from build123d import *

# Parameters (mm, degrees)
BOSS_EXTRU_1_DEPTH      = 23
ENL_V_MAT_EXTRU_1_DEPTH = 21.5
ESQUISSE3_W             = 8.5
ESQUISSE3_H             = 8.4
BOSS_EXTRU_3_DEPTH      = 3.4
BOSS_EXTRU_5_REACH      = 9.309
ESQUISSE4_W             = 1.5
ESQUISSE4_H             = 3.406602833
ESQUISSE23_R            = 1.15
ENL_V_MAT_EXTRU_2_DEPTH = 4
ESQUISSE24_W            = 7
ESQUISSE24_H            = 8.4
BOSS_EXTRU_6_DEPTH      = 3.4
ENL_V_MAT_EXTRU_4_REACH = 77.809
ESQUISSE26_W            = 15.35
ESQUISSE26_H            = 16.4
ESQUISSE27_W            = 1
ESQUISSE27_H            = 17
BOSS_EXTRU_7_DEPTH      = 4
CHANFREIN1_SIZE         = 2
ENL_V_MAT_EXTRU_5_REACH = 76
ESQUISSE28_W            = 4.2
ESQUISSE28_H            = 11.5
ENL_V_MAT_EXTRU_6_REACH = 76
ESQUISSE29_W            = 4.2
ESQUISSE29_H            = 8.5
ESQUISSE30_W            = 13
ESQUISSE30_H            = 4.2
ENL_V_MAT_EXTRU_8_DEPTH = 4
CONG_1_R                = 2


with BuildPart() as part:
    # Esquisse1 → Boss.-Extru.1 (new body)
    with BuildSketch(Plane.XY):
        Polygon((-2.5, -35), (3, -40.809475019), (23, -40.809475019), (28.5, -35), (37, -35), (37, 35), (-37, 35), (-37, -35), align=None)
    extrude(amount=BOSS_EXTRU_1_DEPTH)

    # Esquisse2 → Enlèv. mat.-Extru.1 (cut)
    with BuildSketch(Plane.XY.offset(23)):
        Polygon((-2.5, -33.5), (3, -39.309475019), (23, -39.309475019), (28.5, -33.5), (35.5, -33.5), (35.5, 33.5), (-35.5, 33.5), (-35.5, -33.5), align=None)
    extrude(amount=-ENL_V_MAT_EXTRU_1_DEPTH, mode=Mode.SUBTRACT)

    # Esquisse3 → Boss.-Extru.3 (add)
    with BuildSketch(Plane.XY.offset(1.5)):
        with Locations((31.25, 29.3)):
            Rectangle(ESQUISSE3_W, ESQUISSE3_H)
        with Locations((-31.25, 29.3)):
            Rectangle(ESQUISSE3_W, ESQUISSE3_H)
        with Locations((31.25, -29.3)):
            Rectangle(ESQUISSE3_W, ESQUISSE3_H)
        with Locations((-31.25, -29.3)):
            Rectangle(ESQUISSE3_W, ESQUISSE3_H)
    extrude(amount=BOSS_EXTRU_3_DEPTH)

    # Esquisse4 → Boss.-Extru.5 (add, up to next)
    with BuildSketch(Plane.XZ.offset(33.5), mode=Mode.PRIVATE) as boss_extru_5_sk1:
        with Locations((27.75, 3.196698584)):
            Rectangle(ESQUISSE4_W, ESQUISSE4_H)
    boss_extru_5_tool1 = extrude(boss_extru_5_sk1.sketch, amount=BOSS_EXTRU_5_REACH, mode=Mode.PRIVATE) - part.part
    add(boss_extru_5_tool1.solids().sort_by_distance((27.75, -33.5, 3.196699))[0])

    # Esquisse23 → Enlèv. mat.-Extru.2 (cut)
    with BuildSketch(Plane.XY.offset(4.9)):
        with Locations((31.3, 29.3)):
            Circle(ESQUISSE23_R)
        with Locations((-31.3, 29.3)):
            Circle(ESQUISSE23_R)
        with Locations((31.3, -28.9)):
            Circle(ESQUISSE23_R)
        with Locations((-31.3, -28.9)):
            Circle(ESQUISSE23_R)
    extrude(amount=-ENL_V_MAT_EXTRU_2_DEPTH, mode=Mode.SUBTRACT)

    # Esquisse24 → Boss.-Extru.6 (add)
    with BuildSketch(Plane.XY.offset(1.5)):
        with Locations((-8.3, 29.3)):
            Rectangle(ESQUISSE24_W, ESQUISSE24_H)
        with Locations((-8.3, -29.3)):
            Rectangle(ESQUISSE24_W, ESQUISSE24_H)
    extrude(amount=BOSS_EXTRU_6_DEPTH)

    # Esquisse26 → Enlèv. mat.-Extru.4 (cut, up to next)
    with BuildSketch(Plane.XZ.offset(40.809475019), mode=Mode.PRIVATE) as enl_v_mat_extru_4_sk1:
        with Locations((13, 14.8)):
            Rectangle(ESQUISSE26_W, ESQUISSE26_H)
    enl_v_mat_extru_4_tool1 = extrude(enl_v_mat_extru_4_sk1.sketch, amount=-ENL_V_MAT_EXTRU_4_REACH, mode=Mode.PRIVATE) & part.part
    add(enl_v_mat_extru_4_tool1.solids().sort_by_distance((13, -40.809475, 14.8))[0], mode=Mode.SUBTRACT)

    # Esquisse27 → Boss.-Extru.7 (add)
    with BuildSketch(Plane(origin=(-35.5, 0, 0), x_dir=(0, 0, -1), z_dir=(1, 0, 0))):
        with Locations((-16.9, 3.4)):
            Rectangle(ESQUISSE27_W, ESQUISSE27_H)
    extrude(amount=BOSS_EXTRU_7_DEPTH)

    # Chanfrein1
    chanfrein1_edges = [part.edges().sort_by_distance(p)[0] for p in [
        (-35.5, 3.4, 16.4),
    ]]
    chamfer(chanfrein1_edges, length=CHANFREIN1_SIZE)

    # Esquisse28 → Enlèv. mat.-Extru.5 (cut, up to next)
    with BuildSketch(Plane.ZY.offset(37), mode=Mode.PRIVATE) as enl_v_mat_extru_5_sk1:
        with Locations((20.9, 20.1)):
            Rectangle(ESQUISSE28_W, ESQUISSE28_H)
    enl_v_mat_extru_5_tool1 = extrude(enl_v_mat_extru_5_sk1.sketch, amount=-ENL_V_MAT_EXTRU_5_REACH, mode=Mode.PRIVATE) & part.part
    add(enl_v_mat_extru_5_tool1.solids().sort_by_distance((-37, 20.1, 20.9))[0], mode=Mode.SUBTRACT)

    # Esquisse29 → Enlèv. mat.-Extru.6 (cut, up to next)
    with BuildSketch(Plane.ZY.offset(37), mode=Mode.PRIVATE) as enl_v_mat_extru_6_sk1:
        with Locations((20.9, -8.9)):
            Rectangle(ESQUISSE29_W, ESQUISSE29_H)
    enl_v_mat_extru_6_tool1 = extrude(enl_v_mat_extru_6_sk1.sketch, amount=-ENL_V_MAT_EXTRU_6_REACH, mode=Mode.PRIVATE) & part.part
    add(enl_v_mat_extru_6_tool1.solids().sort_by_distance((-37, -8.9, 20.9))[0], mode=Mode.SUBTRACT)
    # Esquisse29 → Enlèv. mat.-Extru.6 (cut, up to next)
    with BuildSketch(Plane.ZY.offset(37), mode=Mode.PRIVATE) as enl_v_mat_extru_6_sk2:
        with Locations((20.9, -21.5)):
            Rectangle(ESQUISSE29_W, ESQUISSE29_H)
    enl_v_mat_extru_6_tool2 = extrude(enl_v_mat_extru_6_sk2.sketch, amount=-ENL_V_MAT_EXTRU_6_REACH, mode=Mode.PRIVATE) & part.part
    add(enl_v_mat_extru_6_tool2.solids().sort_by_distance((-37, -21.5, 20.9))[0], mode=Mode.SUBTRACT)

    # Esquisse30 → Enlèv. mat.-Extru.8 (cut)
    with BuildSketch(Plane(origin=(0, 35, 0), x_dir=(1, 0, 0), z_dir=(0, 1, 0))):
        with Locations((-17.6, -20.9)):
            Rectangle(ESQUISSE30_W, ESQUISSE30_H)
    extrude(amount=-ENL_V_MAT_EXTRU_8_DEPTH, mode=Mode.SUBTRACT)

    # Congé1
    cong_1_edges = [part.edges().sort_by_distance(p)[0] for p in [
        (28.5, -35, 11.5),
        (23, -40.809475019, 11.5),
        (3, -40.809475019, 11.5),
        (-2.5, -35, 11.5),
        (-37, -35, 11.5),
        (-37, 35, 11.5),
        (37, 35, 11.5),
        (37, -35, 11.5),
        (35.5, 33.5, 13.95),
        (-35.5, 33.5, 13.95),
        (35.5, -33.5, 13.95),
        (-35.5, -33.5, 13.95),
    ]]
    fillet(cong_1_edges, radius=CONG_1_R)


solid = part.part
Could you check a few things on this model? Use its own coordinates, in mm. A direction names the side the tool comes from. Coordinates: 2 decimals unless noted, no trailing zeros. Order: outer loops, then holes, each group sorted by start corner. A loop starts at its lowest first (then second) coordinate and runs counter-clockwise, first axis right, second up.
Q1. Suppose I cut it at A-A on x = 31.3. Please give me the cut outline in (y, z), and give its area (3 significant figures).
Q2. Suppose I cut it at D-D on x = 19.5. Please give me the cut outline in (y, z), and give its area (3 significant figures).
Q3. Which directions (+Z, -Z, +X, -X, +Y, -Y) give clear straight access to the entire face, cutting with the end or side of a thin tool? Please do faces 1 (the flat face through (-37, 0, 11)), 2 (the flat face through (32, -35, 11)), 3 (the flat face through (0.21, -36.36, 12.4)).
Q4. Please list where these lines run through material, in increasing order: L1, parallel to Y at x = 31.3, z = 2.5; L2, parallel to X at y = 30, z = 21.5; L3, parallel to Y at x = -4, z = 16.25.
Q5. Thinking about a two-plate mould opening in X: for faces 4 (the flat face through (0.22, -37.873, 11.339)), 5 (the flat face through (-11.8, -29, 3)), 6 (the flat face through (36, 11, 23)), which applies, released by +X, released by -X, zero draft, split by the parting line, or undercut?
Q6. Will these pins go through, and if not, where does the flat tip stop? pin 1 (2.5 mm diameter, centred on x = 31.3, y = -28.9, fed in from +Z); pin 2 (2 mm diameter, centred on x = -34, y = 2, fed in from +Z); pin 3 (5 mm diameter, centred on x = 11, z = 16, fed in from -Y).
Q7. Suppose I cut it at C-C on y = 24. Please give me the cut outline in (x, z).
Answer:
1. outline: (-35, 0) - (35, 0) - (35, 23) - (33.5, 23) - (33.5, 4.9) - (30.45, 4.9) - (30.45, 0.9) - (28.15, 0.9) - (28.15, 4.9) - (25.1, 4.9) - (25.1, 1.5) - (-25.1, 1.5) - (-25.1, 4.9) - (-27.75, 4.9) - (-27.75, 0.9) - (-30.05, 0.9) - (-30.05, 4.9) - (-33.5, 4.9) - (-33.5, 23) - (-35, 23) - close
1. area: 208 mm2
2. outline: (-40.81, 0) - (35, 0) - (35, 23) - (33.5, 23) - (33.5, 1.5) - (-39.31, 1.5) - (-39.31, 6.6) - (-40.81, 6.6) - close
2. area: 154 mm2
3. face 1: +Z, -Z, -X, +Y, -Y
3. face 2: +Z, -Z, +X, -Y
3. face 3: +Z
4. L1: y = -35 to -30.05, -27.75 to -25.1, 25.1 to 28.15, 30.45 to 35
4. L2: x = -37 to -35.5, 35.5 to 37
4. L3: y = -35 to -33.5, 33.5 to 35
5. face 4: released by -X
5. face 5: undercut
5. face 6: zero draft
6. pin 1: stops at z = 4.9
6. pin 2: stops at z = 17.4
6. pin 3: stops at y = 33.5
7. outline: (-37, 0) - (37, 0) - (37, 23) - (35.5, 23) - (35.5, 1.5) - (-35.5, 1.5) - (-35.5, 18.8) - (-37, 18.8) - close
